Part model, mm, in its own coordinate system. Coordinates: 2 decimals unless noted, no trailing zeros. Loops run counter-clockwise (first coordinate to the right, second up) from the corner with the lowest first, then second, coordinate; pieces in that order, holes last. Notation, with made-up numbers: M 29,19.25 L 75,19.25 A23 ccw 75,50.25 Z; hole C 85,-25.5 d1. An arc over 180 degrees is marked long. Answer as a JSON object with one key per item and string values. Group by question number.
1. Saw through at A-A on x = 0. Write the cut outline in (y, z) (1 decimal).
2. Mould opens along X. For faces 1 (the face through (-3.78, 64.18, -2.9)), 2 (the face through (-1.514, 83.979, -3.773)) say: released by +X, released by -X, zero draft, split by the parting line, or undercut.
3. Drop flat-ended pins along their axis: pin 1 Ø1 at (y, z) = (44.5, 3.5) entering from +X; pin 2 Ø1.9 at (x, y) = (0, 83.5) entering from +Z. Give the stop position or say it passes through.
4. Saw through at B-B on z = 0. Write the cut outline in (x, y) (1 decimal), then the cut area to 3 significant figures.
5. Drill centre lines: L1, parallel to Y at x = 0, z = 3.5 (3 decimals); L2, parallel to Y at x = 1, z = 3.75 (3 decimals); L3, parallel to Z at x = -1.75, y = 91.5. Where is each one in solid material? Low to high.
from build123d import *

# Parameters (mm, degrees)
F0_R        = 4.7625
F1_DEPTH    = 130.175
F3_D        = 6.35
F4_W        = 9.525
F4_H        = 9.525
F5_DEPTH    = 130.175
F7_D        = 3.175
F8_T1_DEPTH = 155.575
F11_D       = 3.175


# Not quite as in the source:
# - a fillet or chamfer that OpenCascade refuses, or shapes differently, is made with other operations: its cross-section is extruded or revolved along the edge and cut away or added


with BuildPart() as f1:
    # F0 (on Front) → F1 (new body)
    with BuildSketch(Plane.XZ):
        Circle(F0_R)
    extrude(amount=-F1_DEPTH)

    # F3 (through all)
    with Locations(Plane.XZ):
        with Locations((0, 0)):
            Hole(F3_D / 2)

    # F11 (through all)
    with Locations(Plane.XY.offset(6.604)):
        with Locations((0, 83.5025), (0, 46.6725)):
            Hole(F11_D / 2)


with BuildPart() as f5:
    # F4 (on Front) → F5 (new body)
    with BuildSketch(Plane.XZ):
        with Locations((196.4227657549, 4.7625)):
            Rectangle(F4_W, F4_H)
    extrude(amount=-F5_DEPTH)

    # F7 (through all)
    with Locations(Plane.XY.offset(9.525)):
        with Locations((196.4227657549, 83.5025), (196.4227657549, 46.6725)):
            Hole(F7_D / 2)

    # F8: fillet of radius 5.08 on 4 edges, made by hand

    # F8_s2 → F8_t1 (cut)
    with BuildSketch(Plane.XZ.offset(-142.875)):
        with BuildLine():
            ThreePointArc((196.1052657549, 9.525), (199.6973682033, 8.0371024484), (201.1852657549, 4.445))
            Line((201.1852657549, 4.445), (201.1852657549, 9.525))
            Line((201.1852657549, 9.525), (196.1052657549, 9.525))
        make_face()
        with BuildLine():
            ThreePointArc((191.6602657549, 4.445), (193.1481633065, 8.0371024484), (196.7402657549, 9.525))
            Line((196.7402657549, 9.525), (191.6602657549, 9.525))
            Line((191.6602657549, 9.525), (191.6602657549, 4.445))
        make_face()
        with BuildLine():
            ThreePointArc((196.1052657549, 0), (199.6973682033, 1.4878975516), (201.1852657549, 5.08))
            Line((201.1852657549, 5.08), (201.1852657549, 0))
            Line((201.1852657549, 0), (196.1052657549, 0))
        make_face()
        with BuildLine():
            ThreePointArc((191.6602657549, 5.08), (193.1481633065, 1.4878975516), (196.7402657549, 0))
            Line((196.7402657549, 0), (191.6602657549, 0))
            Line((191.6602657549, 0), (191.6602657549, 5.08))
        make_face()
    extrude(amount=F8_T1_DEPTH, mode=Mode.SUBTRACT)


solid = f1.part
Outcome:
{
 "1": {"outline": "M 0,-4.8 L 45.1,-4.8 L 45.1,-3.2 L 0,-3.2 Z; M 0,3.2 L 45.1,3.2 L 45.1,4.8 L 0,4.8 Z; M 48.3,-4.8 L 81.9,-4.8 L 81.9,-3.2 L 48.3,-3.2 Z; M 48.3,3.2 L 81.9,3.2 L 81.9,4.8 L 48.3,4.8 Z; M 85.1,-4.8 L 130.2,-4.8 L 130.2,-3.2 L 85.1,-3.2 Z; M 85.1,3.2 L 130.2,3.2 L 130.2,4.8 L 85.1,4.8 Z"},
 "2": {"face 1": "split by the parting line", "face 2": "undercut"},
 "3": {"pin 1": "stops at x = 3.7", "pin 2": "passes through"},
 "4": {"outline": "M -4.8,0 L -3.2,0 L -3.2,130.2 L -4.8,130.2 Z; M 3.2,0 L 4.8,0 L 4.8,130.2 L 3.2,130.2 Z", "area": "413 mm²"},
 "5": {"L1": "y = 0 to 45.085, 48.26 to 81.915, 85.09 to 130.175", "L2": "y = 0 to 45.44, 47.905 to 82.27, 84.735 to 130.175", "L3": "z = -4.43 to -2.65, 2.65 to 4.43"}
}
